Check sheet for the modelled part. Datum: model origin and axes. Units: mm. A direction names the side the tool comes from. Round coordinates to 2 decimals unless told otherwise and drop trailing zeros. Loops run counter-clockwise (first coordinate to the right, second up) from the corner with the lowest first, then second, coordinate; pieces in that order, holes last. Notation, with made-up numbers: (4.5, 71.25) -> (46.5, 71.25) arc R24 ccw to (46.5, 91.25) -> close; hole circle Ø11 at (-30.75, 61.5). An arc over 180 degrees is marked (long way). One line per item, written item: value. Start each with the question number.
1. Set-up check for faces 4 (the face through (-91.699, 19, 20)), 5 (the face through (-69, 36, -21.476)), 6 (the face through (-65, 37, 3)), 7 (the face through (-89.699, 17, 4)), 8 (the face through (-99, 1, 9.254)): record each of +Z, -Z, +X, -X, +Y, -Y from which the full face is reachable in a straight line by a thin tool's end or side.
2. Cross-section at C-C on z = 22.5. Record the cut outline in (x, y).
3. Go/stop test with flat-tipped pins: pin 1 (8 mm diameter, centred on y = 25, z = 0, fed in from -X); pin 2 (8 mm diameter, centred on y = -1, z = -23, fed in from -X); pin 3 (3 mm diameter, centred on x = -37, z = -19, fed in from -Y); pin 4 (12 mm diameter, centred on y = -5.5, z = -28.5, fed in from -X). Record where each tip stops, or that it passes through.
4. Material ranges on L1, parallel to X at y = -1, z = 0.5; L2, parallel to X at y = 7.5, z = 17.5; L3, parallel to Y at x = 14.5, z = 20.5, recorded low to high.
5. Cross-section at A-A on x = -28.5. Record the cut outline in (y, z).
6. Release check for a two-part mould opening along X. For faces 1 (the face through (-91.699, 19, -6)), 2 (the face through (-79.91, 36.01, -12.62)), 3 (the face through (-37.699, 19, 4)) record: +X half, -X half, draft (parallel to the pull), parting line (faces both ways), or undercut.
from build123d import *

# Parameters (mm, degrees)
SKETCH2_W                = 130
SKETCH2_H                = 70
BOSS_EXTRUDE1_DEPTH      = 2
SKETCH3_W                = 54
SKETCH3_H                = 70
BOSS_EXTRUDE2_DEPTH      = 35
SKETCH4_W                = 50
SKETCH4_H                = 70
CUT_EXTRUDE2_DEPTH       = 33
CUT_EXTRUDE2_DEPTH_BACK  = 2
SKETCH6_W                = 50
SKETCH6_H                = 2
CUT_EXTRUDE3_DEPTH       = 33
SKETCH7_W                = 70
SKETCH7_H                = 20
CUT_EXTRUDE4_DEPTH       = 40
M3_CLEARANCE_HOLE4_D     = 3.4
M3_CLEARANCE_HOLE4_DEPTH = 3.5
M3_CLEARANCE_HOLE4_TIP   = 1.021463052
SKETCH21_W               = 15
SKETCH21_H               = 15
REVOLVE1_ANGLE           = 60
SKETCH22_W               = 15
SKETCH22_H               = 2.941288486
CUT_EXTRUDE6_DEPTH       = 55
SKETCH23_W               = 8
SKETCH23_H               = 16.328711514
CUT_EXTRUDE7_DEPTH       = 55


with BuildPart() as part:
    # Sketch2 → Boss-Extrude1 (new body)
    with BuildSketch(Plane(origin=(0, 0, 0), x_dir=(1, 0, 0), z_dir=(0, 1, 0))):
        with Locations((-41.699117153, 6.475560132)):
            Rectangle(SKETCH2_W, SKETCH2_H)
    extrude(amount=BOSS_EXTRUDE1_DEPTH)

    # Sketch3 → Boss-Extrude2 (add)
    with BuildSketch(Plane(origin=(0, 2, 0), x_dir=(1, 0, 0), z_dir=(0, 1, 0))):
        with Locations((-64.699117153, 6.461257978)):
            Rectangle(SKETCH3_W, SKETCH3_H)
    extrude(amount=BOSS_EXTRUDE2_DEPTH)

    # Sketch4 → Cut-Extrude2 (cut, two sides)
    with BuildSketch(Plane(origin=(0, 2, 0), x_dir=(1, 0, 0), z_dir=(0, 1, 0))) as cut_extrude2_sk:
        with Locations((-64.699117153, 6.461257978)):
            Rectangle(SKETCH4_W, SKETCH4_H)
    extrude(amount=CUT_EXTRUDE2_DEPTH, mode=Mode.SUBTRACT)
    extrude(cut_extrude2_sk.sketch, amount=-CUT_EXTRUDE2_DEPTH_BACK, mode=Mode.SUBTRACT)

    # Sketch6 → Cut-Extrude3 (cut)
    with BuildSketch(Plane(origin=(0, 0, -41.475560132), x_dir=(-1, 0, 0), z_dir=(0, 0, -1))):
        with Locations((64.699117153, 1)):
            Rectangle(SKETCH6_W, SKETCH6_H)
    extrude(amount=-CUT_EXTRUDE3_DEPTH, mode=Mode.SUBTRACT)

    # Sketch7 → Cut-Extrude4 (cut)
    with BuildSketch(Plane.XZ):
        with Locations((-71.699117153, -31.475560132)):
            Rectangle(SKETCH7_W, SKETCH7_H)
    extrude(amount=-CUT_EXTRUDE4_DEPTH, mode=Mode.SUBTRACT)

    # M3 Clearance Hole4
    with Locations(Plane(origin=(0, 35, 0), x_dir=(-1, 0, 0), z_dir=(0, -1, 0))):
        with Locations((49.339561588, -18.538742022), (49.699117153, 11.475560132), (78.653715997, -18.538742022), (78.653715997, 11.475560132)):
            Hole(M3_CLEARANCE_HOLE4_D / 2, depth=M3_CLEARANCE_HOLE4_DEPTH)
            with Locations((0, 0, -(M3_CLEARANCE_HOLE4_DEPTH + M3_CLEARANCE_HOLE4_TIP / 2))):  # 118° drill point
                Cone(0, M3_CLEARANCE_HOLE4_D / 2, M3_CLEARANCE_HOLE4_TIP, mode=Mode.SUBTRACT)

    # Sketch21 → Revolve1 (revolve)
    with BuildSketch(Plane.XZ):
        with Locations((-22.811286853, 1.754439868)):
            Rectangle(SKETCH21_W, SKETCH21_H)
    revolve1 = revolve(axis=Axis((-30.311286853, 0, 9.254439868), (-1, 0, 0)), revolution_arc=REVOLVE1_ANGLE)

    # Sketch22 → Cut-Extrude6 (cut)
    with BuildSketch(Plane.XZ):
        with Locations((-22.811286853, 10.725084111)):
            Rectangle(SKETCH22_W, SKETCH22_H)
    cut_extrude6 = extrude(amount=-CUT_EXTRUDE6_DEPTH, mode=Mode.SUBTRACT)

    # Sketch23 → Cut-Extrude7 (cut)
    with BuildSketch(Plane.XZ):
        with Locations((-22.811286853, 20.360084111)):
            Rectangle(SKETCH23_W, SKETCH23_H)
    cut_extrude7 = extrude(amount=-CUT_EXTRUDE7_DEPTH, mode=Mode.SUBTRACT)

    # Mirror1: Revolve1 across plane
    add(revolve1.mirror(Plane.ZY.offset(60.999117153)))

    # Mirror2: Cut-Extrude6, Cut-Extrude7 across plane
    add(cut_extrude6.mirror(Plane.ZY.offset(60.999117153)), mode=Mode.SUBTRACT)
    add(cut_extrude7.mirror(Plane.ZY.offset(60.999117153)), mode=Mode.SUBTRACT)


solid = part.part
Taken from the geometry:
1. face 4: +Z, -Z, -X, +Y
1. face 5: -Z, -X, +Y, -Y
1. face 6: +Z, -Z, +X, -X, +Y
1. face 7: +Z, -Z, -Y
1. face 8: +Y, -Y
2. outline: (-106.7, 0) -> (-103.19, 0) -> (-103.19, 2) -> (-106.7, 2) -> close; (-95.19, 0) -> (-89.7, 0) -> (-89.7, 35) -> (-39.7, 35) -> (-39.7, 0) -> (-26.81, 0) -> (-26.81, 2) -> (-37.7, 2) -> (-37.7, 37) -> (-91.7, 37) -> (-91.7, 2) -> (-95.19, 2) -> close; (-18.81, 0) -> (23.3, 0) -> (23.3, 2) -> (-18.81, 2) -> close
3. pin 1: stops at x = -91.7
3. pin 2: stops at x = -106.7
3. pin 3: stops at y = 0
3. pin 4: stops at x = -36.7
4. L1: x = -106.69 to -91.69, -30.31 to -15.31
4. L2: x = -91.7 to -89.7, -39.7 to -37.7
4. L3: y = 0 to 2
5. outline: (-12.99, 1.75) arc R15 ccw to (0, -5.75) -> (0, -41.48) -> (2, -41.48) -> (2, 9.25) -> (0, 9.25) -> close; (0, 12.2) -> (2, 12.2) -> (2, 28.52) -> (0, 28.52) -> close
6. face 1: -X half
6. face 2: undercut
6. face 3: +X half
